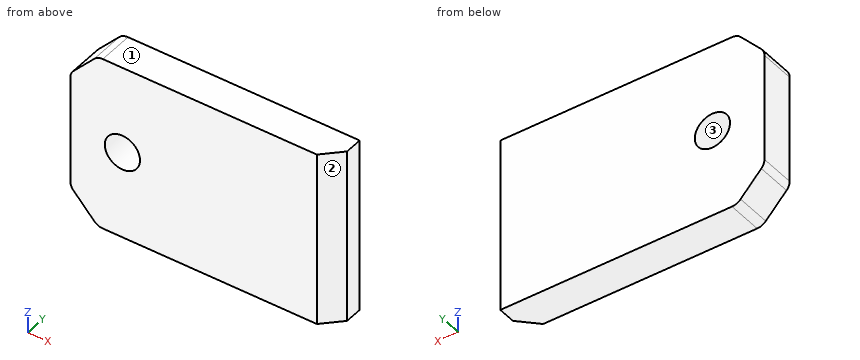
from build123d import *

# Parameters (mm, degrees)
SKETCH_1_W          = 30
SKETCH_1_H          = 6
EXTRUDE_1_DEPTH     = 45
CHAMFER_1_SIZE      = 3
SKETCH_2_R          = 3
CUT_EXTRUDE_1_DEPTH = 55.415071442
CHAMFER_2_SIZE      = 5
CHAMFER_2_SIZE2     = 4.662575431
FILLET_1_R          = 2


with BuildPart() as part:
    # Эскиз1 → Вытянуть1 (new body)
    with BuildSketch(Plane(origin=(0, 0, 0), x_dir=(0, 0, -1), z_dir=(1, 0, 0))):
        with Locations((15, -3)):
            Rectangle(SKETCH_1_W, SKETCH_1_H)
    extrude(amount=EXTRUDE_1_DEPTH)

    # Фаска1
    chamfer_1_edges = [part.edges().sort_by_distance(p)[0] for p in [
        (45, -6, -15),
    ]]
    chamfer(chamfer_1_edges, length=CHAMFER_1_SIZE)

    # Эскиз2 → Вырез-Вытянуть1 (cut, through all)
    with BuildSketch(Plane(origin=(0, 0, 0), x_dir=(-1, 0, 0), z_dir=(0, 1, 0))):
        with Locations(Location((-8.86993337, -14.999999492, 0), (0, 0, 90))):
            Circle(SKETCH_2_R)
    extrude(amount=-CUT_EXTRUDE_1_DEPTH, mode=Mode.SUBTRACT)

    # Фаска2
    chamfer_2_edges = [part.edges().sort_by_distance(p)[0] for p in [
        (0, -3, -30),
        (0, -3, 0),
    ]]
    chamfer_2_side = [part.faces().sort_by_distance(p)[0] for p in [
        (0, -3, -15),
    ]]
    chamfer(chamfer_2_edges, length=CHAMFER_2_SIZE, length2=CHAMFER_2_SIZE2, reference=chamfer_2_side[0])

    # Скругление1
    fillet_1_edges = [part.edges().sort_by_distance(p)[0] for p in [
        (4.662575431, -3, -30),
        (0, -3, -5),
        (0, -3, -25),
        (4.662575431, -3, 0),
    ]]
    fillet(fillet_1_edges, radius=FILLET_1_R)


solid = part.part
Work out the finished part from the listing and answer in its coordinate system (mm). Face numbers are marked on the shaded views. Give positions to 0.01 mm unless a question says otherwise; leave off trailing zeros. Order: outer loops, then holes, each group sorted by start corner. A loop starts at its lowest first (then second) coordinate and runs counter-clockwise, first axis right, second up. Notation, with made-up numbers: (24.25, 15.25) -> (64.25, 15.25) arc R22 ccw to (64.25, 27.25) -> close; hole circle Ø7 at (27, 0.5). An arc over 180 degrees is marked (long way). Answer as a JSON object with one key per item and string values. Group by question number.
1. Section C-C on x = 6.5 is taken. Determine the outline of the cut face in (y, z).
2. Consider line 1 along X through (y, z) = (-1.95, -15); line 2 along Z through (x, y) = (8, -5.5); line 3 along X through (y, z) = (-4.55, -15). Determine where each line is inside the solid, lowest interval first. Write a range as [from, to].
3. Flat-ended cylindrical pins translate along their axes: pin 1 Ø1.5 at (y, z) = (-5, -23.5) entering from +X; pin 2 Ø5.5 at (x, z) = (8.87, -15) entering from -Y. Find the tip coordinate at first contact, or state that the pin passes through.
4. The mould has two halves that part along X. Classify the marked faces 1, 2 and 3: released by +X, released by -X, zero draft, split by the parting line, or undercut.
5. Section A-A on z = -15 is taken. Determine the outline of the cut face in (x, y), plus the area to 4 significant figures.
6. Section B-B on y = -2.25 is taken. Determine the outline of the cut face in (x, z), plus the area to 3 significant figures.
7. Section D-D on z = -19 is taken. Determine the outline of the cut face in (x, y).
Result sheet:
{
 "1": {"outline": "(-6, -30) -> (0, -30) -> (0, -16.84) -> (-6, -16.84) -> close; (-6, -13.16) -> (0, -13.16) -> (0, 0) -> (-6, 0) -> close"},
 "2": {"line 1": "x = [0, 5.87], [11.87, 45]", "line 2": "z = [-30, -17.87], [-12.13, 0]", "line 3": "x = [0, 5.87], [11.87, 43.45]"},
 "3": {"pin 1": "stops at x = 43.75", "pin 2": "passes through"},
 "4": {"face 1": "zero draft", "face 2": "released by +X", "face 3": "undercut"},
 "5": {"outline": "(0, -6) -> (5.87, -6) -> (5.87, 0) -> (0, 0) -> close; (11.87, -6) -> (42, -6) -> (45, -3) -> (45, 0) -> (11.87, 0) -> close", "area": "229.5 mm^2"},
 "6": {"outline": "(0, -24.21) arc R2 ccw to (0.54, -25.58) -> (4.07, -29.36) arc R2 ccw to (5.53, -30) -> (45, -30) -> (45, 0) -> (5.53, 0) arc R2 ccw to (4.07, -0.64) -> (0.54, -4.42) arc R2 ccw to (0, -5.79) -> close; hole circle Ø6 at (8.87, -15)", "area": "1,300 mm^2"},
 "7": {"outline": "(0, -6) -> (42, -6) -> (45, -3) -> (45, 0) -> (0, 0) -> close"}
}
